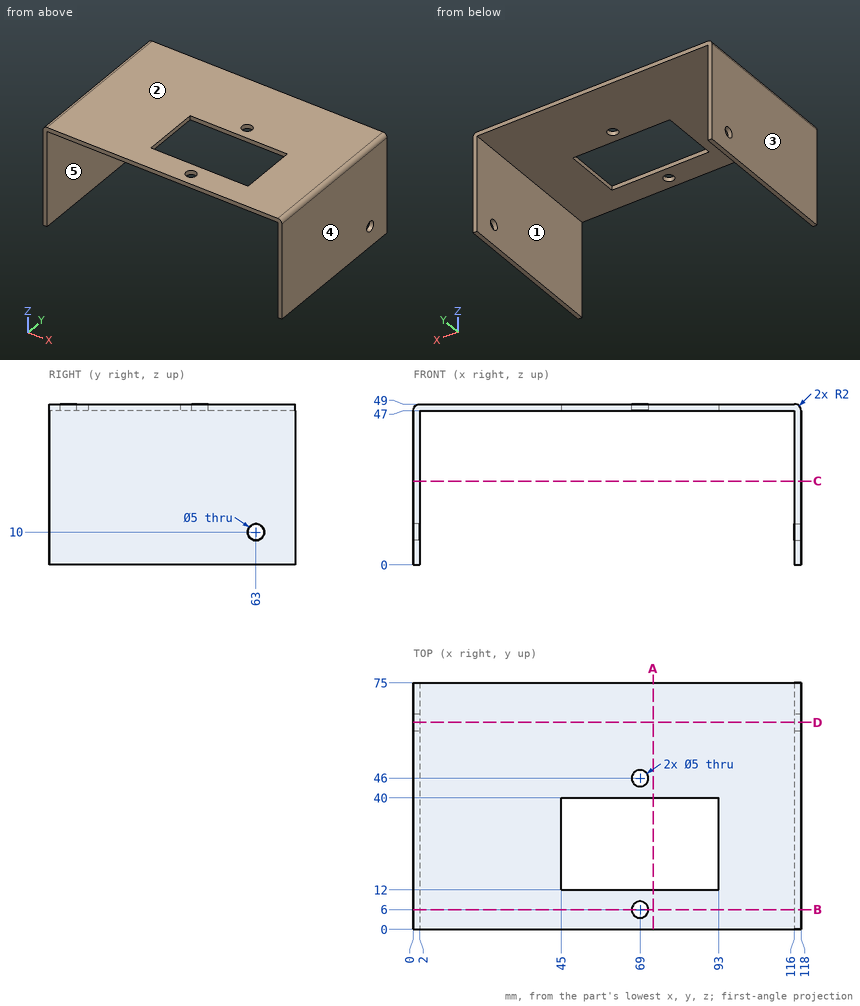
Input: dimensioned drawing with shaded views. Units: mm. Origin: part minimum x, y, z. A direction names the side the tool comes from. Round coordinates to 2 decimals unless told otherwise and drop trailing zeros. Loops run counter-clockwise (first coordinate to the right, second up) from the corner with the lowest first, then second, coordinate; pieces in that order, holes last. Notation, with made-up numbers: (21, 59) -> (42, 59) arc R25 cw to (42, 88) -> close; hole circle Ø3 at (-14, 28.5). An arc over 180 degrees is marked (long way). Use one line per item in the form item = value. Start each with the question number.
1) Access query for the marked faces 4 and 5. Directions: +Z, -Z, +X, -X, +Y, -Y. A direction counts if a zero-diameter tool reaches every point of the face in a straight line with its end or side. Return the directions, or none.
2) Draft query along X for the marked faces 1, 2 and 3. Return one class per face: released by +X, released by -X, zero draft, split by the parting line, or undercut.
3) Section D-D on y = 63. Output: boundary loops of the cut face in (x, z), then the cut area to 3 significant figures.
4) Section A-A on x = 73. Output: boundary loops of the cut face in (y, z), then the cut area to 3 significant figures.
5) Section C-C on z = 25.5. Output: boundary loops of the cut face in (x, y).
6) Line query: L1, parallel to X at y = 33, z = 23; L2, parallel to Z at x = 0.7, y = 63; L3, parallel to Z at x = 19, y = 51. Output: solid intervals per line, ascending.
7) First-contact query: P1, Ø6, axis at x = 69, y = 6, coming from the -Z side; P2, Ø1.6, axis at y = 28, z = 48, coming from the -X side; P3, Ø3, axis at y = 63, z = 10, coming from the -X side. Flat tips, straight axial feed; report the tip coordinate or a pass-through.
8) Section B-B on y = 6. Output: boundary loops of the cut face in (x, z), then the cut area to 3 significant figures.
Response:
q1.face_4 = +Z, -Z, +X, +Y, -Y
q1.face_5 = -Z, +Y, -Y
q2.face_1 = undercut
q2.face_2 = zero draft
q2.face_3 = released by -X
q3.outline = (0, 0) -> (2, 0) -> (2, 7.5) -> (0, 7.5) -> close; (0, 12.5) -> (2, 12.5) -> (2, 47) -> (116, 47) -> (116, 12.5) -> (118, 12.5) -> (118, 47) arc R2 ccw to (116, 49) -> (2, 49) arc R2 ccw to (0, 47) -> close; (116, 0) -> (118, 0) -> (118, 7.5) -> (116, 7.5) -> close
q3.area = 402 mm^2
q4.outline = (0, 47) -> (12, 47) -> (12, 49) -> (0, 49) -> close; (40, 47) -> (75, 47) -> (75, 49) -> (40, 49) -> close
q4.area = 94.0 mm^2
q5.outline = (0, 0) -> (2, 0) -> (2, 75) -> (0, 75) -> close; (116, 0) -> (118, 0) -> (118, 75) -> (116, 75) -> close
q6.L1 = 0 to 2, 116 to 118
q6.L2 = 0 to 7.5, 12.5 to 48.52
q6.L3 = 47 to 49
q7.P1 = 47
q7.P2 = 0.01
q7.P3 = through
q8.outline = (0, 0) -> (2, 0) -> (2, 47) -> (66.5, 47) -> (66.5, 49) -> (2, 49) arc R2 ccw to (0, 47) -> close; (71.5, 47) -> (116, 47) -> (116, 0) -> (118, 0) -> (118, 47) arc R2 ccw to (116, 49) -> (71.5, 49) -> close
q8.area = 412 mm^2
